```python
from build123d import *

# Parameters (mm, degrees)
F0_R     = 25.4
F3_R     = 18.6067290317
F8_DEPTH = 5.08
F9_DEPTH = 5.08


# Not quite as in the source:
# - a feature of the source that left no trace in its solid (it failed there, or was rolled back) is left out


with BuildPart() as f4:
    # F0 (on Top) → F4 section 0
    with BuildSketch(Plane.XY):
        Circle(F0_R)
    # F3 (on plane+point) → F4 section 1
    with BuildSketch(Plane.XY.offset(-19.05)):
        Circle(F3_R)
    loft()

    # F5 (on face) → F8 (cut)
    with BuildSketch(Plane(origin=(0, 0, -19.05), x_dir=(1, 0, 0), z_dir=(0, 0, -1))):
        with BuildLine():
            Line((18.5089529757, 1.905), (2.0125971848, 1.905))
            Line((2.0125971848, 1.905), (2.0125971848, 0))
            Line((2.0125971848, 0), (2.0125971848, -1.905))
            Line((2.0125971848, -1.905), (18.5089529757, -1.905))
            ThreePointArc((18.5089529757, -1.905), (18.5822689403, -0.9537537886), (18.6067290317, 0))
            ThreePointArc((18.6067290317, 0), (18.5822689403, 0.9537537886), (18.5089529757, 1.905))
        make_face()
    extrude(amount=-F8_DEPTH, mode=Mode.SUBTRACT)

    # F5 (on face) → F9 (cut)
    with BuildSketch(Plane(origin=(0, 0, -19.05), x_dir=(1, 0, 0), z_dir=(0, 0, -1))):
        with BuildLine():
            Line((26.4462942035, 1.905), (18.5089529757, 1.905))
            ThreePointArc((18.5089529757, 1.905), (18.5822689403, 0.9537537886), (18.6067290317, 0))
            ThreePointArc((18.6067290317, 0), (18.5822689403, -0.9537537886), (18.5089529757, -1.905))
            Line((18.5089529757, -1.905), (26.4462942035, -1.905))
            Line((26.4462942035, -1.905), (26.4462942035, 1.905))
        make_face()
    extrude(amount=-F9_DEPTH, mode=Mode.SUBTRACT)


solid = f4.part
```
Can you work these out from the model? Positions are in its coordinate system, mm. A direction names the side the tool comes from. Coordinates: 2 decimals unless noted, no trailing zeros. Loops run counter-clockwise (first coordinate to the right, second up) from the corner with the lowest first, then second, coordinate; pieces in that order, holes last. Notation, with made-up numbers: (-27, -27) - (29, -27) arc R13 ccw to (29, -14) - close; hole circle Ø2 at (-19, 19). An arc over 180 degrees is marked (long way). Answer as CSV lines item,"result". Start each with the question number.
1) Suppose I cut it at C-C (z = -11.25). Please give me the cut outline in (x, y).
2) Suppose I cut it at B-B (z = -7.75). Please give me the cut outline in (x, y), plus the area to 3 significant figures.
3) Thinking about a two-plate mould opening in Y: for faces 1 (the flat face through (11, -1.905, -17)), 2 (the conical face through (-4.269, -19.223, -16.008)), 3 (the flat face through (0, 0, -19.05)), which applies, pulls with the +Y half, pulls with the -Y half, needs draft (parallel to the pull), parting line crosses it, or undercut?
4) I need wall thicknesses on line 1 (Y direction, x = 6.5, z = -16.5) (3 decimals); line 2 (Z direction, x = 14.5, y = 13.5); line 3 (X direction, y = -6, z = -3.5). Which ranges of each line are inside material? Lowest first, please. Write a range as from..to.
5) Suppose I cut it at A-A (x = 0). Please give me the cut outline in (y, z).
6) Which directions (+Z, -Z, +X, -X, +Y, -Y) give clear straight access to the entire face, cutting with the end or side of a thin tool? Please do faces 4 (the flat face through (11, 0, -13.97)), 5 (the flat face through (0, 0, 0)).
7) For pin 1 (1.5 mm diameter, centred on y = -2, z = -13, fed in from +X); pin 2 (1.1 mm diameter, centred on x = 14, y = 1, fed in from -Z); pin 3 (1.5 mm diameter, centred on x = 20, y = -13, fed in from +Z); pin 4 (3 mm diameter, centred on y = 0, z = -16.5, fed in from +X), each with a flat end and sliding along its axis, tell me the tip position at first contact or that it passes through.
Check result:
1,outline,"circle Ø42.78 at (0, 0)"
2,outline,"circle Ø45.27 at (0, 0)"
2,area,"1,610 mm²"
3,face 1,"undercut"
3,face 2,"parting line crosses it"
3,face 3,"needs draft"
4,line 1,"y = -18.402..-1.905, 1.905..18.402"
4,line 2,"z = -15.67..0"
4,line 3,"x = -23.39..23.39"
5,outline,"(-25.4, 0) - (-18.61, -19.05) - (18.61, -19.05) - (25.4, 0) - close"
6,face 4,"-Z, +X"
6,face 5,"+Z, +X, -X, +Y, -Y"
7,pin 1,"stops at x = 20.94"
7,pin 2,"stops at z = -13.97"
7,pin 3,"stops at z = 0"
7,pin 4,"stops at x = 2.01"
